Input: dimensioned drawing with shaded views. Units: mm. Origin: part minimum x, y, z. A direction names the side the tool comes from. Round coordinates to 2 decimals unless told otherwise and drop trailing zeros. Order: outer loops, then holes, each group sorted by start corner. A loop starts at its lowest first (then second) coordinate and runs counter-clockwise, first axis right, second up. Notation, with made-up numbers: (84, 14) - (104, 14) arc R25 cw to (104, 49) - close; hole circle Ø1 at (13.5, -30.5). An arc over 180 degrees is marked (long way). Put each result on its own line as item: value. Start each with the question number.
(1) Section D-D (z = 24). Output: boundary loops of the cut face in (x, y), and give its area (3 significant figures).
(2) Section A-A (z = 29). Output: boundary loops of the cut face in (x, y), and give its area (3 significant figures).
(3) Pull-direction query (Y, two-part tool) for the marked faces 3, 4, 5 and 6; classes: released by +Y, released by -Y, zero draft, split by the parting line, or undercut.
(4) Section B-B (y = 20.5). Output: boundary loops of the cut face in (x, z) (1 decimal), and give its area (3 significant figures).
(5) Access query for the marked faces 1 and 2. Directions: +Z, -Z, +X, -X, +Y, -Y. A direction counts if a zero-diameter tool reaches every point of the face in a straight line with its end or side. Return the directions, or none.
(6) Material intervals for L1, parallel to Y at x = 13.25, z = 26.5; L2, parallel to X at y = 11.5, z = 23.5; L3, parallel to Z at x = 10, y = 32.5, sorted ascending. Write a range as [from, to].
(7) Pin query (flat end, axial travel): P1, Ø10.5, axis at x = 4, y = 19.5, coming from the +Z side; P2, Ø4, axis at y = 22, z = 24, coming from the -X side. Return the tip coordinate at first contact, or that it passes through.
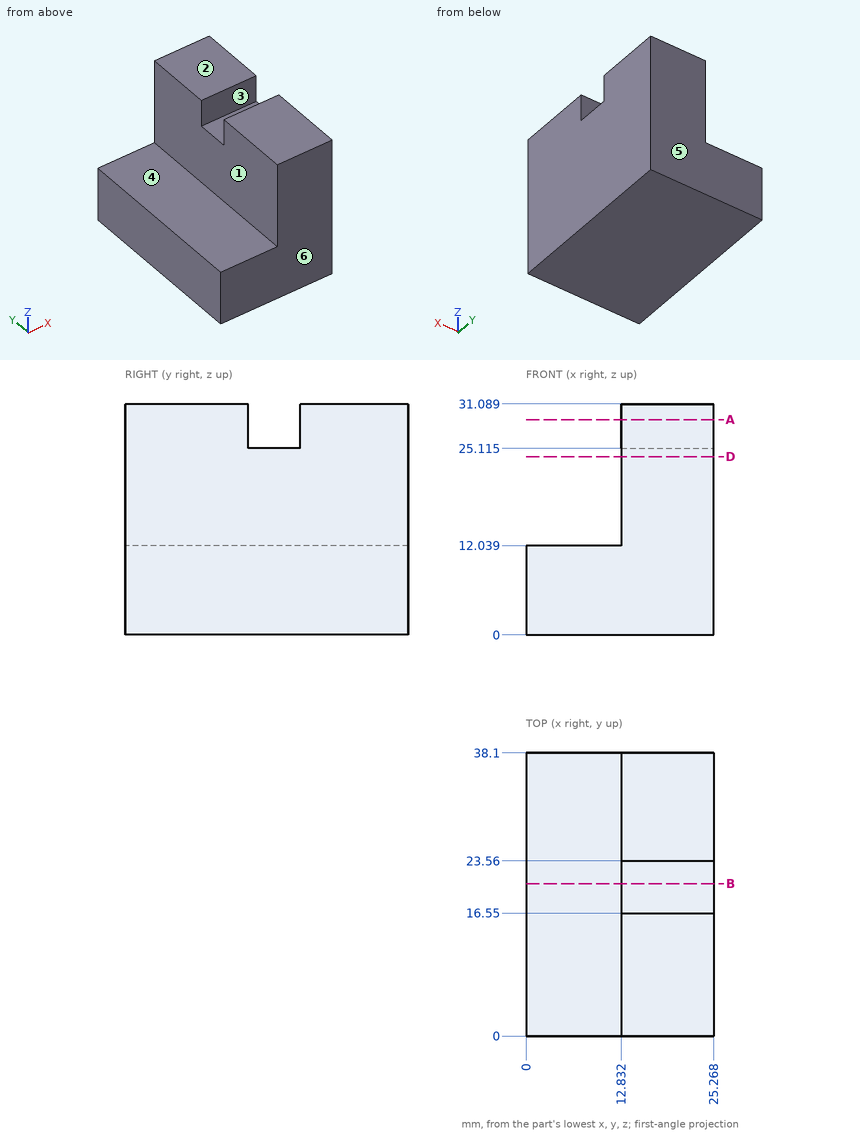
Checks:
1. outline: (12.83, 0) - (25.27, 0) - (25.27, 38.1) - (12.83, 38.1) - close
1. area: 474 mm²
2. outline: (12.83, 0) - (25.27, 0) - (25.27, 16.55) - (12.83, 16.55) - close; (12.83, 23.56) - (25.27, 23.56) - (25.27, 38.1) - (12.83, 38.1) - close
2. area: 387 mm²
3. face 3: undercut
3. face 4: zero draft
3. face 5: released by +Y
3. face 6: released by -Y
4. outline: (0, 0) - (25.3, 0) - (25.3, 25.1) - (12.8, 25.1) - (12.8, 12) - (0, 12) - close
4. area: 467 mm²
5. face 1: +Z, -X, +Y, -Y
5. face 2: +Z, +X, -X, +Y, -Y
6. L1: y = [0, 16.55], [23.56, 38.1]
6. L2: x = [12.83, 25.27]
6. L3: z = [0, 12.04]
7. P1: stops at z = 12.04
7. P2: stops at x = 12.83
